The listing builds one solid part. Answer for the finished solid, in the listing's coordinates (mm). A direction names the side the tool comes from. Coordinates: 2 decimals unless noted, no trailing zeros. Loops run counter-clockwise (first coordinate to the right, second up) from the corner with the lowest first, then second, coordinate; pieces in that order, holes last. Notation, with made-up numbers: (71, -13) - (129, -13) arc R23 cw to (129, 14) - close; hole circle Ø8 at (73, -21.5). An arc over 180 degrees is marked (long way). Return JSON: item names as keys, results as strings. Group by question number.
1. The mould has two halves that part along X. Classify faces 6 (the face through (151, -22, 0)), 7 (the face through (95.143, -33, 0)), 8 (the face through (165.33, -11.15, -6.75)): pulls with the +X half, pulls with the -X half, needs draft (parallel to the pull), parting line crosses it, or undercut.
2. Section A-A (x = 0) is taken. Write down the section's boundary in (y, z) (3 decimals), and give its area (3 significant figures).
3. Which of the six approach directions +Z, -Z, +X, -X, +Y, -Y give full straight-line access (tool end or side, diameter ignored) to faces 1 (the face through (38, -59, -16)), 2 (the face through (76, 0, 1)), 3 (the face through (123, -22, 41)), 4 (the face through (-38, -59, 16)), 5 (the face through (151, -33, -25))?
4. Find the intervals of material crossed by line 1 along Z through (x, y) = (162.5, -31); line 2 along X through (y, z) = (-20, -5.5); line 3 along Y through (x, z) = (81.5, 3), in increasing order.
5. Section C-C (y = -6.5) is taken. Write down the section's boundary in (x, z) (3 decimals), and give its area (3 significant figures).
6. Section B-B (y = -29) is taken. Write down the section's boundary in (x, z) (3 decimals).
7. Section D-D (z = -33.5) is taken. Write down the section's boundary in (x, y), and give its area (3 significant figures).
8. Each of these flat-tipped pins is pushed along its axis until it touches: P1, Ø5, axis at y = -46, z = 13, coming from the -X side; P2, Ø11, axis at x = 173.5, y = -35.5, coming from the +Z side; P3, Ø3, axis at x = -40, y = -59, coming from the -Z side. Where does it stop, or does it pass through?
```python
from build123d import *

# Parameters (mm, degrees)
F0_R     = 28.575
F1_DEPTH = 64
F2_DEPTH = 44
F3_R     = 11.1
F4_DEPTH = 44.001
F3_W     = 114
F3_H     = 50
F5_DEPTH = 22
F7_DEPTH = 10
F9_DEPTH = 95.001


with BuildPart() as f1:
    # F0 (on Front) → F1 (new body)
    with BuildSketch(Plane.XZ):
        with BuildLine():
            ThreePointArc((35.142567, -41), (49.05965, -22.564368), (54, 0))
            ThreePointArc((54, 0), (49.05965, 22.564368), (35.142567, 41))
            ThreePointArc((35.142567, 41), (-54, 0), (35.142567, -41))
        make_face()
        Circle(F0_R, mode=Mode.SUBTRACT)
    extrude(amount=F1_DEPTH)

    # F0 (on Front) → F2 (join)
    with BuildSketch(Plane.XZ):
        with BuildLine():
            ThreePointArc((35.142567, 41), (49.05965, 22.564368), (54, 0))
            ThreePointArc((54, 0), (49.05965, -22.564368), (35.142567, -41))
            Line((35.142567, -41), (209.142567, -41))
            Line((209.142567, -41), (209.142567, 41))
            Line((209.142567, 41), (35.142567, 41))
        make_face()
    extrude(amount=F2_DEPTH)

    # F3 (on face) → F4 (cut, through all)
    with BuildSketch(Plane.XZ.offset(44)):
        with Locations((174.142567, 0)):
            Circle(F3_R)
        with Locations((124.142567, 0)):
            Circle(F3_R)
    extrude(amount=-F4_DEPTH, mode=Mode.SUBTRACT)

    # F3 (on face) → F5 (cut)
    with BuildSketch(Plane.XZ.offset(44)):
        with Locations((152.142567, 0)):
            Rectangle(F3_W, F3_H)
        with Locations((124.142567, 0)):
            Circle(F3_R, mode=Mode.SUBTRACT)
        with Locations((174.142567, 0)):
            Circle(F3_R, mode=Mode.SUBTRACT)
    extrude(amount=-F5_DEPTH, mode=Mode.SUBTRACT)

    # F6 (on face) → F7 (cut)
    with BuildSketch(Plane.XZ.offset(64)):
        with BuildLine():
            ThreePointArc((51.575188, 16), (0, 54), (-51.575188, 16))
            Line((-51.575188, 16), (-23.675528, 16))
            ThreePointArc((-23.675528, 16), (0, 28.575), (23.675528, 16))
            Line((23.675528, 16), (51.575188, 16))
        make_face()
        with BuildLine():
            Line((-23.675528, -16), (-51.575188, -16))
            ThreePointArc((-51.575188, -16), (0, -54), (51.575188, -16))
            Line((51.575188, -16), (23.675528, -16))
            ThreePointArc((23.675528, -16), (0, -28.575), (-23.675528, -16))
        make_face()
    extrude(amount=-F7_DEPTH, mode=Mode.SUBTRACT)

    # F8 (on face) → F9 (cut, through all)
    with BuildSketch(Plane.XY.offset(41)):
        Polygon((197.142567, -44), (209.142567, -44), (209.142567, -32), align=None)
    extrude(amount=-F9_DEPTH, mode=Mode.SUBTRACT)


solid = f1.part
```
The answers:
{
 "1": {"face 6": "needs draft", "face 7": "pulls with the +X half", "face 8": "undercut"},
 "2": {"outline": "(-54, -54) - (0, -54) - (0, -28.575) - (-54, -28.575) - close; (-54, 28.575) - (0, 28.575) - (0, 54) - (-54, 54) - close", "area": "2,750 mm2"},
 "3": {"face 1": "-Z, +X, -X, -Y", "face 2": "+Z, -Z, +X, -X, +Y", "face 3": "+Z, +X, +Y, -Y", "face 4": "+Z, +X, -X, -Y", "face 5": "+X, -Y"},
 "4": {"line 1": "z = -41 to -25, 25 to 41", "line 2": "x = -53.72 to -28.04, 28.04 to 114.5, 133.78 to 164.5, 183.78 to 209.14", "line 3": "y = -44 to 0"},
 "5": {"outline": "(35.143, -41) - (209.143, -41) - (209.143, 41) - (35.143, 41) arc R54 ccw (long way) to start; hole circle Ø57.15 at (0, 0); hole circle Ø22.2 at (124.143, 0); hole circle Ø22.2 at (174.143, 0)", "area": "19,000 mm2"},
 "6": {"outline": "(35.143, -41) - (209.143, -41) - (209.143, -25) - (95.143, -25) - (95.143, 25) - (209.143, 25) - (209.143, 41) - (35.143, 41) arc R54 ccw (long way) to start; hole circle Ø57.15 at (0, 0)"},
 "7": {"outline": "(-42.35, -54) - (42.35, -54) - (42.35, -44) - (197.14, -44) - (209.14, -32) - (209.14, 0) - (-42.35, 0) - close", "area": "11,800 mm2"},
 "8": {"P1": "stops at x = -52.97", "P2": "stops at z = 41", "P3": "stops at z = -16"}
}
